Autodesk Inventor part; units mm, degrees
ref_plane "YZ Plane" through (0, 0, 0) normal (1, 0, 0) x (0, 1, 0)
ref_plane "XZ Plane" through (0, 0, 0) normal (0, 1, 0) x (-1, 0, 0)
ref_plane "XY Plane" through (0, 0, 0) normal (0, 0, 1) x (1, 0, 0)
sketch "Sketch1" plane through (0, 0, 0) normal (0, 1, 0) x (-1, 0, 0)
  circle A0 centre (0, 0) radius 10.9855
  line L0 (12.7, -25.4) -> (-12.7, -25.4)
  line L1 (-12.7, -25.4) -> (-12.7, 25.4)
  line L2 (-12.7, 25.4) -> (12.7, 25.4)
  line L3 (12.7, 25.4) -> (12.7, -25.4)
  line L4 (12.7, -25.4) -> (-12.7, 25.4) construction
  line L5 (-12.7, -25.4) -> (12.7, 25.4) construction
  circle A1 centre (0, 0) radius 19.05
  circle A2 centre (-6.35, -19.05) radius 2.159
  circle A3 centre (6.35, -19.05) radius 2.159
  circle A4 centre (-6.35, 19.05) radius 2.159
  circle A5 centre (6.35, 19.05) radius 2.159
  point P0 (-12.7, -14.199)
  point P1 (12.7, -14.199)
  point P2 (12.7, 14.199)
  point P3 (-12.7, 14.199)
  dimension "d0" = 21.971
  dimension "d1" = 25.4
  dimension "d2" = 50.8
  dimension "d3" = 38.1
  dimension "d4" = 4.318
  dimension "d5" = 6.35
  dimension "d6" = 6.35
  dimension "d9" = 12.7
  dimension "d12" = 38.1
extrude "Extrusion1" add sketch "Sketch1" along normal blind 1.5875 contours L0 L1 A1 A2 A3 L3 | A1 A3 A2 L1 A4 A5 L3 | L3 A1 | A1 L1 | A1 A5 A4 L1 L2 L3
fillet "Fillet1" radius 31.75 4 edges at (12.7, 0.7937, 14.199) (12.7, 0.7937, -14.199) (-12.7, 0.7937, -14.199) (-12.7, 0.7937, 14.199)
properties part number "ball bearing holder" material "Acetal Resin, Black"
Verification items for the finished model (mm, model axes). Round coordinates to 2 decimals unless told otherwise and drop trailing zeros. Order: outer loops, then holes, each group sorted by start corner. A loop starts at its lowest first (then second) coordinate and runs counter-clockwise, first axis right, second up.
1) Cross-section at D-D, the plane x = 6.35. Record the cut outline in (y, z), plus the area to 3 significant figures.
Geometry says:
outline: (0, -25.4) - (1.59, -25.4) - (1.59, -21.21) - (0, -21.21) - close; (0, -16.89) - (1.59, -16.89) - (1.59, -8.96) - (0, -8.96) - close; (0, 8.96) - (1.59, 8.96) - (1.59, 16.89) - (0, 16.89) - close; (0, 21.21) - (1.59, 21.21) - (1.59, 25.4) - (0, 25.4) - close
area: 38.5 mm2
2) Cross-section at B-B, the plane z = 4.5. Record the cut outline in (x, y), plus the area to 3 significant figures.
Geometry says:
outline: (-18.51, 0) - (-10.02, 0) - (-10.02, 1.59) - (-18.51, 1.59) - close; (10.02, 0) - (18.51, 0) - (18.51, 1.59) - (10.02, 1.59) - close
area: 27.0 mm2
3) Material ranges on line 1 (X direction, y = 0.5, z = -19.05); line 2 (Z direction, x = 0, y = 0.85); line 3 (X direction, y = 0.6, z = -20), recorded low to high.
Geometry says:
line 1: x = -13.19 to -8.51, -4.19 to 4.19, 8.51 to 13.19
line 2: z = -25.4 to -10.99, 10.99 to 25.4
line 3: x = -13.03 to -8.29, -4.41 to 4.41, 8.29 to 13.03
4) Cross-section at C-C, the plane y = 0.35. Record the cut outline in (x, z).
Geometry says:
outline: (-16.67, -9.22) arc R31.75 cw to (-12.7, -24.59) - (-12.7, -25.4) - (12.7, -25.4) - (12.7, -24.59) arc R31.75 cw to (16.67, -9.22) arc R19.05 ccw to (16.67, 9.22) arc R31.75 cw to (12.7, 24.59) - (12.7, 25.4) - (-12.7, 25.4) - (-12.7, 24.59) arc R31.75 cw to (-16.67, 9.22) arc R19.05 ccw to start; hole circle Ø21.97 at (0, 0); hole circle Ø4.32 at (-6.35, -19.05); hole circle Ø4.32 at (-6.35, 19.05); hole circle Ø4.32 at (6.35, -19.05); hole circle Ø4.32 at (6.35, 19.05)
5) Depth check by flat-ended pin: pin 1 (0.6 mm diameter, centred on y = 1, z = 25, fed in from -X); pin 2 (0.6 mm diameter, centred on y = 1, z = 25, fed in from +X); pin 3 (3.5 mm diameter, centred on x = 6.35, z = -19.05, fed in from -Y). Enter the tip coordinate at first touch or a pass-through.
Geometry says:
pin 1: stops at x = -12.7
pin 2: stops at x = 12.7
pin 3: passes through
6) Draft check along X on faces 1 (the cylindrical face through (-5.882, 0.783, 21.158)), 2 (the cylindrical face through (-19.05, 0.78, 0.13)), 3 (the flat face through (0, 1, 25.4)), 4 (the cylindrical face through (13.68, 0.8, -16.76)). Enter one of: +X half, -X half, draft (parallel to the pull), parting line (faces both ways), or undercut.
Geometry says:
face 1: undercut
face 2: -X half
face 3: draft
face 4: +X half
7) Cross-section at A-A, the plane x = 0. Record the cut outline in (y, z), plus the area to 3 significant figures.
Geometry says:
outline: (0, -25.4) - (1.59, -25.4) - (1.59, -10.99) - (0, -10.99) - close; (0, 10.99) - (1.59, 10.99) - (1.59, 25.4) - (0, 25.4) - close
area: 45.8 mm2
